The figure shows three views and two pictorial views of one solid part (mm, origin at its lowest corner). Answer the questions. A direction names the side the tool comes from. Round coordinates to 2 decimals unless told otherwise and drop trailing zeros. Order: outer loops, then holes, each group sorted by start corner. A loop starts at its lowest first (then second) coordinate and runs counter-clockwise, first axis right, second up. Notation, with made-up numbers: (86, -39.5) - (113, -39.5) arc R19 cw to (113, -11.5) - close; hole circle Ø11 at (89.25, 59). An arc over 180 degrees is marked (long way). Write item = value, one per line.
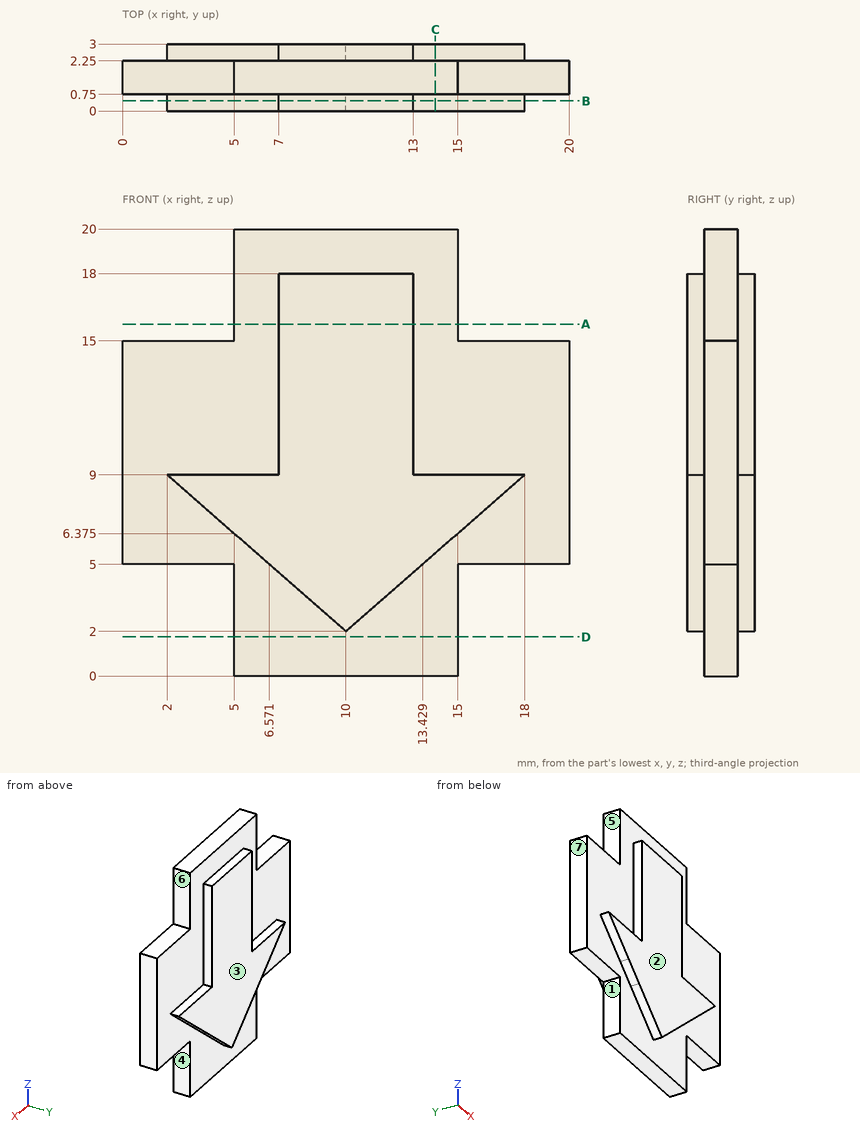
Q1. For the marked faces 4, 5, 6 and 7, determine the directions among +Z, -Z, +X, -X, +Y, -Y from which every point of the face is accessible in a straight line to the end or side of a thin tool.
Model answer:
face_4 = -Z, +X, +Y, -Y
face_5 = +Z, -X, +Y, -Y
face_6 = +Z, +X, +Y, -Y
face_7 = +Z, -Z, -X, +Y, -Y
Q2. Section A-A on z = 15.75 is taken. Determine the outline of the cut face in (x, y), then the cut area to 3 significant figures.
Model answer:
outline = (5, 0.75) - (7, 0.75) - (7, 0) - (13, 0) - (13, 0.75) - (15, 0.75) - (15, 2.25) - (13, 2.25) - (13, 3) - (7, 3) - (7, 2.25) - (5, 2.25) - close
area = 24.0 mm^2
Q3. Find the intervals of material crossed by line 1 (X direction, y = 0.5, z = 13.75); line 2 (Z direction, x = 18.75, y = 2.15); line 3 (Y direction, x = 14.5, z = 1.75), in increasing order. Write a range as from..to.
Model answer:
line_1 = 7..13
line_2 = 5..15
line_3 = 0.75..2.25
Q4. Section B-B on y = 0.45 is taken. Determine the outline of the cut face in (x, z) (1 decimal).
Model answer:
outline = (2, 9) - (10, 2) - (18, 9) - (13, 9) - (13, 18) - (7, 18) - (7, 9) - close
Q5. Determine the mould class of the marked faces 1, 2 and 3 for opening direction Y: released by +Y, released by -Y, zero draft, split by the parting line, or undercut.
Model answer:
face_1 = zero draft
face_2 = released by -Y
face_3 = released by +Y
Q6. Section D-D on z = 1.75 is taken. Determine the outline of the cut face in (x, y).
Model answer:
outline = (5, 0.75) - (15, 0.75) - (15, 2.25) - (5, 2.25) - close
Q7. Flat-ended cylindrical pins translate along their axes: P1, Ø0.8, axis at y = 1.5, z = 2, coming from the +X side; P2, Ø1.6, axis at x = 18.5, y = 1.5, coming from the -Z side; P3, Ø2, axis at x = 4.5, z = 12.5, coming from the -Y side. Find the tip coordinate at first contact, or state that the pin passes through.
Model answer:
P1 = 15
P2 = 5
P3 = 0.75
Q8. Section C-C on x = 14 is taken. Determine the outline of the cut face in (y, z).
Model answer:
outline = (0, 5.5) - (0.75, 5.5) - (0.75, 0) - (2.25, 0) - (2.25, 5.5) - (3, 5.5) - (3, 9) - (2.25, 9) - (2.25, 20) - (0.75, 20) - (0.75, 9) - (0, 9) - close
